Autodesk Inventor part; units mm, degrees
ref_plane "YZ Plane" through (0, 0, 0) normal (1, 0, 0) x (0, 1, 0)
ref_plane "XZ Plane" through (0, 0, 0) normal (0, 1, 0) x (-1, 0, 0)
ref_plane "XY Plane" through (0, 0, 0) normal (0, 0, 1) x (1, 0, 0)
sketch "Sketch1" plane through (0, 0, 0) normal (0, 0, 1) x (1, 0, 0)
  point P0 (0, 0)
sketch "Sketch2" plane through (0, 0, 0) normal (0, 0, 1) x (1, 0, 0)
  line L0 (127, 965.2) -> (341.7889, 965.2) construction
  line L1 (279.4, 965.2) -> (279.4, 0) construction
  line L2 (279.4, 482.6) -> (-286.2053, 482.6) construction
  line L3 (127, 965.2) -> (0, 745.2295)
  line L4 (431.8, 965.2) -> (558.8, 745.2295)
  line L5 (127, 0) -> (0, 219.9705)
  line L6 (431.8, 0) -> (558.8, 219.9705)
  line L7 (0, 219.9705) -> (0, 745.2295)
  line L8 (558.8, 745.2295) -> (558.8, 219.9705)
  line L9 (0, 745.2295) -> (127, 965.2)
  line L10 (0, 745.2295) -> (0, 219.9705)
  line L11 (0, 219.9705) -> (127, 0)
  line L12 (431.8, 0) -> (558.8, 219.9705)
  line L13 (558.8, 219.9705) -> (558.8, 745.2295)
  line L14 (558.8, 745.2295) -> (431.8, 965.2)
  line L15 (127, 0) -> (431.8, 0)
  line L16 (431.8, 965.2) -> (127, 965.2)
  point P0 (0, 0)
  point P1 (341.7889, 0)
  dimension "d3" = 152.4
  dimension "d4" = 152.4
  dimension "d10" = 525.2591
  dimension "d11" = 525.2591
  dimension "d15" = 304.8
  dimension "d16" = 219.9704
extrude "Extrusion1" add sketch "Sketch2" along normal blind 152.4
properties part number "4901BaseSolidGeometry"
Check sheet for the modelled part. Datum: model origin and axes. Units: mm. Coordinates: 2 decimals unless noted, no trailing zeros. Loops run counter-clockwise (first coordinate to the right, second up) from the corner with the lowest first, then second, coordinate; pieces in that order, holes last. Notation, with made-up numbers: (12.25, -32) -> (53.25, -32) arc R21 ccw to (53.25, -12) -> close; hole circle Ø6 at (11, 18). An arc over 180 degrees is marked (long way). Write item = value, one per line. Start each with the question number.
1. Section check C-C on y = 73. Record the cut outline in (x, z).
2. Depth check by flat-ended pin: P1, Ø3, axis at x = 213, y = 723, coming from the -Z side; P2, Ø2, axis at x = 81, z = 40.5, coming from the -Y side. Enter the tip coordinate at first touch or a pass-through.
3. Material ranges on line 1 (X direction, y = 755.5, z = 87); line 2 (Y direction, x = 514.5, z = 18.5); line 3 (Y direction, x = 43.5, z = 79.5), recorded low to high.
4. Section check B-B on x = 47. Record the cut outline in (y, z).
5. Section check A-A on z = 32. Record the cut outline in (x, y), then the cut area to 3 significant figures.
Responses:
q1.outline = (84.85, 0) -> (473.95, 0) -> (473.95, 152.4) -> (84.85, 152.4) -> close
q2.P1 = 0
q2.P2 = 77.94
q3.line_1 = 5.93 to 552.87
q3.line_2 = 143.24 to 821.96
q3.line_3 = 144.63 to 820.57
q4.outline = (138.56, 0) -> (826.64, 0) -> (826.64, 152.4) -> (138.56, 152.4) -> close
q5.outline = (0, 219.97) -> (127, 0) -> (431.8, 0) -> (558.8, 219.97) -> (558.8, 745.23) -> (431.8, 965.2) -> (127, 965.2) -> (0, 745.23) -> close
q5.area = 483,000 mm2
